Here's how the part is built. I have some questions about the finished solid (model axes, mm). Face numbers are marked on the shaded views. A direction names the side the tool comes from. Round coordinates to 2 decimals unless told otherwise and drop trailing zeros. Loops run counter-clockwise (first coordinate to the right, second up) from the corner with the lowest first, then second, coordinate; pieces in that order, holes last. Notation, with made-up numbers: M 56.25,-39 L 65.25,-39 A11 cw 65.25,-23 Z; hole C -28,-23 d6. An arc over 180 degrees is marked long. Use a Markdown table: item, result.
```python
from build123d import *

# Parameters (mm, degrees)
BOSS_EXTRUDE1_DEPTH = 21
BOSS_EXTRUDE2_DEPTH = 2


with BuildPart() as part:
    # Sketch1 → Boss-Extrude1 (new body)
    with BuildSketch(Plane(origin=(0, 0, 0), x_dir=(1, 0, 0), z_dir=(0, 1, 0))):
        with BuildLine():
            Line((2.265430343, 29.914341466), (2.274223615, 29.914341466))
            Line((2.274223615, 29.914341466), (2.274223615, 41.938382264))
            ThreePointArc((2.274223615, 41.938382264), (-0.004403071, -41.999999769), (-2.265430343, 41.938858179))
            Line((-2.265430343, 41.938858179), (-2.265430343, 29.914341466))
            ThreePointArc((-2.265430343, 29.914341466), (0, -30), (2.265430343, 29.914341466))
        make_face()
    extrude(amount=BOSS_EXTRUDE1_DEPTH)

    # Boss-Extrude2: read off the stored shape, not the designer's step
    # Boss-Extrude2 outline → Boss-Extrude2 (add)
    with BuildSketch(Plane(origin=(0, 21, 0), x_dir=(1, 0, 0), z_dir=(0, 1, 0))):
        with BuildLine():
            ThreePointArc((-2.265430343, 44.942939661), (-0.004402235, -44.999999785), (2.274223615, 44.942495558))
            Line((2.274223615, 44.942495558), (2.274223325, 29.913674269))
            ThreePointArc((2.274223325, 29.913674269), (-0.004409129, -29.999999676), (-2.265430343, 29.914341466))
            Line((-2.265430343, 29.914341466), (-2.265430343, 44.942939661))
        make_face()
    extrude(amount=BOSS_EXTRUDE2_DEPTH)


solid = part.part
```
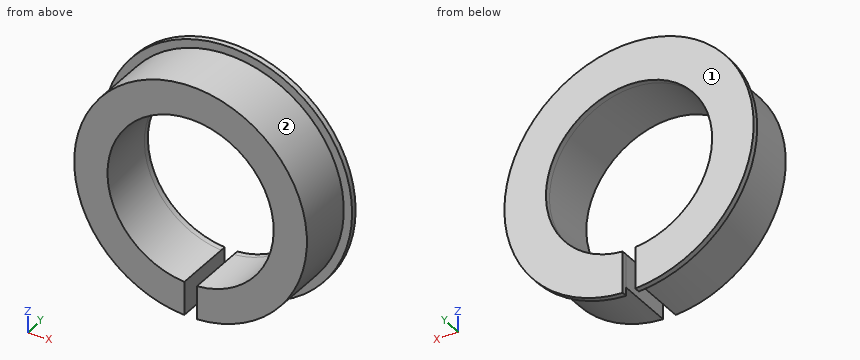
Q1. I need wall thicknesses on line 1 (X direction, y = 22, z = 0); line 2 (Z direction, x = 0, y = 22); line 3 (Z direction, x = 0, y = 10.75). Which ranges of each line are inside material? Lowest first, please. Write a range as from..to.
Return value:
| item | result |
|---|---|
| line 1 | x = -45..-30, 30..45 |
| line 2 | z = 30..45 |
| line 3 | z = 30..42 |
Q2. Imagine slicing it at B-B, the plane x = -9. Please give me the cut outline in (y, z).
Return value:
| item | result |
|---|---|
| outline | M 0,-41.02 L 21,-41.02 L 21,-44.09 L 23,-44.09 L 23,-28.62 L 0,-28.62 Z; M 0,28.62 L 23,28.62 L 23,44.09 L 21,44.09 L 21,41.02 L 0,41.02 Z |
Q3. Imagine slicing it at A-A, the plane z = 0. Please give me the cut outline in (x, y), then the cut area to 3 significant figures.
Return value:
| item | result |
|---|---|
| outline | M -45,21 L -42,21 L -42,0 L -30,0 L -30,23 L -45,23 Z; M 30,0 L 42,0 L 42,21 L 45,21 L 45,23 L 30,23 Z |
| area | 564 mm^2 |
Q4. Imagine slicing it at D-D, the plane x = -32.5. Please give me the cut outline in (y, z).
Return value:
| item | result |
|---|---|
| outline | M 0,-26.6 L 21,-26.6 L 21,-31.12 L 23,-31.12 L 23,31.12 L 21,31.12 L 21,26.6 L 0,26.6 Z |
Q5. Will these pins go through, and if not, where does the flat tip stop? P1, Ø6, axis at y = 13.5, z = -35, coming from the -X side; P2, Ø10, axis at x = 0, y = 7.5, coming from the +Z side; P3, Ø12, axis at x = -0.5, y = 17.5, coming from the +Z side.
Return value:
| item | result |
|---|---|
| P1 | stops at x = -27.2 |
| P2 | stops at z = 42 |
| P3 | stops at z = 45 |
Q6. For the marked faces 1 and 2, which set-ups out of +Z, -Z, +X, -X, +Y, -Y let a thin tool reach every point of the face, with its end or its side?
Return value:
| item | result |
|---|---|
| face 1 | +Z, -Z, +X, -X, +Y |
| face 2 | -Y |
